Autodesk Inventor part; units mm, degrees
ref_plane "YZ Plane" through (0, 0, 0) normal (1, 0, 0) x (0, 1, 0)
ref_plane "XZ Plane" through (0, 0, 0) normal (0, 1, 0) x (-1, 0, 0)
ref_plane "XY Plane" through (0, 0, 0) normal (0, 0, 1) x (1, 0, 0)
sketch "Эскиз1" plane through (0, 0, 0) normal (0, 0, 1) x (1, 0, 0)
  line L0 (125, -28.5) -> (-125, -28.5)
  line L1 (-125, -28.5) -> (-125, 28.5)
  line L2 (-125, 28.5) -> (125, 28.5)
  line L3 (125, 28.5) -> (125, -28.5)
  line L4 (125, -28.5) -> (-125, 28.5) construction
  line L5 (-125, -28.5) -> (125, 28.5) construction
  line L6 (-125, 28.5) -> (125, 28.5)
  line L7 (125, 11.5) -> (-125, 11.5)
  line L8 (-125, 11.5) -> (-125, 28.5)
  line L9 (-125, 11.5) -> (125, 11.5)
  line L10 (125, 11.5) -> (125, -8.5)
  line L11 (125, -8.5) -> (-125, -8.5)
  line L12 (-125, -8.5) -> (-125, 11.5)
  line L13 (-125, -8.5) -> (125, -8.5)
  line L14 (125, -8.5) -> (125, -25.5)
  line L15 (125, -25.5) -> (-125, -25.5)
  line L16 (-125, -25.5) -> (-125, -8.5)
  line L17 (-125, 28.5) -> (125, 28.5)
  line L18 (125, 25.5) -> (-125, 25.5)
  line L19 (-125, 25.5) -> (-125, 28.5)
  line L20 (-125, 28.5) -> (-111, 28.5)
  line L21 (-111, 28.5) -> (-111, 25.5)
  line L22 (-111, 25.5) -> (-125, 25.5)
  line L23 (-125, 25.5) -> (-125, 28.5)
  line L24 (-111, 25.5) -> (-99, 25.5)
  line L25 (-99, 25.5) -> (-99, 28.5)
  line L26 (-99, 28.5) -> (-111, 28.5)
  line L27 (-111, 28.5) -> (-111, 25.5)
  line L28 (-99, 28.5) -> (-87, 28.5)
  line L29 (-87, 28.5) -> (-87, 25.5)
  line L30 (-87, 25.5) -> (-99, 25.5)
  line L31 (-99, 25.5) -> (-99, 28.5)
  line L32 (-111, 28.5) -> (-106.35, 28.5)
  line L33 (-106.35, 28.5) -> (-103.65, 28.5)
  line L34 (-103.65, 28.5) -> (-103.65, 8.5)
  line L35 (-103.65, 8.5) -> (-106.35, 8.5)
  line L36 (-106.35, 8.5) -> (-106.35, 28.5)
  line L37 (-106.35, 25.5) -> (-107.45, 25.5)
  line L38 (-107.45, 22.5) -> (-106.35, 22.5)
  line L39 (-106.35, 22.5) -> (-106.35, 25.5)
  line L40 (-107.45, 22.5) -> (-102.55, 22.5)
  line L41 (-102.55, 22.5) -> (-102.55, 20.6)
  line L42 (-102.55, 20.6) -> (-107.45, 20.6)
  line L43 (-107.45, 20.6) -> (-107.45, 22.5)
  line L44 (125, -28.5) -> (125, 28.5)
  line L45 (111, 28.5) -> (111, 25.5)
  line L46 (99, 25.5) -> (99, 28.5)
  line L47 (87, 28.5) -> (87, 25.5)
  line L48 (103.65, 28.5) -> (103.65, 8.5)
  line L49 (103.65, 8.5) -> (106.35, 8.5)
  line L50 (106.35, 8.5) -> (106.35, 28.5)
  line L51 (106.35, 22.5) -> (106.35, 25.5)
  line L52 (107.45, 22.5) -> (102.55, 22.5)
  line L53 (102.55, 22.5) -> (102.55, 20.6)
  line L54 (102.55, 20.6) -> (107.45, 20.6)
  line L55 (107.45, 20.6) -> (107.45, 22.5)
  line L56 (-125, 11.5) -> (-96, 11.5)
  line L57 (-96, 11.5) -> (-96, -8.5)
  line L58 (-96, -8.5) -> (-125, -8.5)
  line L59 (-125, -8.5) -> (-125, 11.5)
  line L60 (-96, -8.5) -> (-67, -8.5)
  line L61 (-67, -8.5) -> (-67, 11.5)
  line L62 (-67, 11.5) -> (-96, 11.5)
  line L63 (-96, 11.5) -> (-96, -8.5)
  line L64 (-96, 1.5) -> (-93, 1.5)
  line L65 (-67, 1.5) -> (-70, 1.5)
  circle A0 centre (-70, 1.5) radius 1.5
  circle A1 centre (-93, 1.5) radius 1.5
  circle A2 centre (70, 1.5) radius 1.5
  circle A3 centre (93, 1.5) radius 1.5
  line L66 (-125, 28.5) -> (-122, 28.5)
  line L67 (-126, 8.5) -> (-125, 28.5)
  line L68 (-126, -3.5) -> (-126, 8.5)
  line L69 (-126, 1.15) -> (-126, 3.85)
  line L70 (-125, 28.5) -> (-123, 28.5)
  line L71 (-123, 28.5) -> (-123, 8.5)
  line L72 (-123, 8.5) -> (-125, 8.5)
  line L73 (-125, 8.5) -> (-125, 28.5)
  line L74 (-123, 8.5) -> (-126, 8.5)
  line L75 (-126, 8.5) -> (-126, -3.5)
  line L76 (-126, -3.5) -> (-123, -3.5)
  line L77 (-123, -3.5) -> (-123, 8.5)
  line L78 (-123, 28.5) -> (-120, 28.5)
  line L79 (-120, 28.5) -> (-120, -3.5)
  line L80 (-120, -3.5) -> (-123, -3.5)
  line L81 (-123, -3.5) -> (-123, 28.5)
  line L82 (-123, 8.5) -> (-120, 8.5)
  line L83 (-120, 8.5) -> (-120, -3.5)
  line L84 (-120, -3.5) -> (-123, -3.5)
  line L85 (-123, -3.5) -> (-123, 8.5)
  line L86 (-123, 8.5) -> (-123, 3.85)
  line L87 (-123, 3.85) -> (-103, 3.85)
  line L88 (-103, 3.85) -> (-103, 1.15)
  line L89 (-103, 1.15) -> (-123, 1.15)
  line L90 (-123, 1.15) -> (-123, 3.85)
  line L91 (-120, 1.15) -> (-117, 1.15)
  line L92 (-117, 1.15) -> (-117, 0.05)
  line L93 (-117, 0.05) -> (-120, 0.05)
  line L94 (-120, 0.05) -> (-120, 1.15)
  line L95 (-117, 0.05) -> (-115.1, 0.05)
  line L96 (-115.1, 0.05) -> (-115.1, 4.95)
  line L97 (-115.1, 4.95) -> (-117, 4.95)
  line L98 (-117, 4.95) -> (-117, 0.05)
  line L99 (123, 3.85) -> (103, 3.85)
  line L100 (103, 3.85) -> (103, 1.15)
  line L101 (103, 1.15) -> (123, 1.15)
  line L102 (120, 1.15) -> (117, 1.15)
  line L103 (117, 0.05) -> (115.1, 0.05)
  line L104 (115.1, 0.05) -> (115.1, 4.95)
  line L105 (115.1, 4.95) -> (117, 4.95)
  line L106 (117, 4.95) -> (117, 0.05)
  line L107 (126, -3.5) -> (123, -3.5)
  line L108 (120, 28.5) -> (120, -3.5)
  line L109 (120, -3.5) -> (123, -3.5)
  line L110 (123, -3.5) -> (123, 28.5)
  line L111 (123, 8.5) -> (125, 8.5)
  line L112 (123, 8.5) -> (120, 8.5)
  line L113 (-123, -3.5) -> (-125, -3.5)
  line L114 (-125, -3.5) -> (-125, -28.5)
  line L115 (-125, -28.5) -> (-123, -28.5)
  line L116 (-123, -28.5) -> (-123, -3.5)
  line L117 (123, -3.5) -> (125, -3.5)
  line L118 (125, -3.5) -> (125, -28.5)
  line L119 (125, -28.5) -> (123, -28.5)
  line L120 (123, -28.5) -> (123, -3.5)
  line L121 (-67, -8.5) -> (-14.5, -8.5)
  line L122 (-14.5, -28.5) -> (-67, -28.5)
  line L123 (-40.75, -28.5) -> (-33.75, -28.5)
  circle A4 centre (-33.75, -21.5) radius 1.5
  circle A5 centre (-47.75, -21.5) radius 1.5
  circle A6 centre (33.75, -21.5) radius 1.5
  circle A7 centre (47.75, -21.5) radius 1.5
  line L124 (-33.75, -25.5) -> (-47.75, -25.5)
  line L125 (-47.75, -28.5) -> (-33.75, -28.5)
  line L126 (-40.75, -28.5) -> (-28.75, -28.5)
  line L127 (-28.75, -28.5) -> (-28.75, -25.5)
  line L128 (-28.75, -25.5) -> (-40.75, -25.5)
  line L129 (-40.75, -28.5) -> (-52.75, -28.5)
  line L130 (-52.75, -28.5) -> (-52.75, -25.5)
  line L131 (-52.75, -25.5) -> (-40.75, -25.5)
  line L132 (-40.75, -25.5) -> (-40.75, -28.5)
  line L133 (28.75, -28.5) -> (28.75, -25.5)
  line L134 (52.75, -28.5) -> (52.75, -25.5)
  line L135 (52.5, -17.5) -> (-52.5, -17.5)
  line L136 (-52.5, -17.5) -> (-52.5, 17.5)
  line L137 (-52.5, 17.5) -> (52.5, 17.5)
  line L138 (52.5, 17.5) -> (52.5, -17.5)
  line L139 (52.5, -17.5) -> (-52.5, 17.5) construction
  line L140 (-52.5, -17.5) -> (52.5, 17.5) construction
  line L141 (15, 14.5) -> (-15, 14.5)
  line L142 (-15, 14.5) -> (-15, 20.5)
  line L143 (-15, 20.5) -> (15, 20.5)
  line L144 (15, 20.5) -> (15, 14.5)
  line L145 (15, 14.5) -> (-15, 20.5) construction
  line L146 (-15, 14.5) -> (15, 20.5) construction
  line L147 (15, -20.5) -> (-15, -20.5)
  line L148 (-15, -20.5) -> (-15, -14.5)
  line L149 (-15, -14.5) -> (15, -14.5)
  line L150 (15, -14.5) -> (15, -20.5)
  line L151 (15, -20.5) -> (-15, -14.5) construction
  line L152 (-15, -20.5) -> (15, -14.5) construction
  line L153 (0, 0) -> (-36, 0)
  line L154 (-36, 0) -> (-36, 28.5)
  line L155 (-36, 28.5) -> (0, 28.5)
  line L156 (0, 28.5) -> (0, 0)
  line L157 (0, 0) -> (47, 0)
  line L158 (47, 0) -> (47, 28.5)
  line L159 (47, 28.5) -> (0, 28.5)
  line L160 (0, 28.5) -> (0, 0)
  line L161 (-36, 28.5) -> (-33, 28.5)
  line L162 (-33, 28.5) -> (-33, 25.5)
  line L163 (-33, 25.5) -> (-36, 25.5)
  line L164 (-36, 25.5) -> (-36, 28.5)
  line L165 (-36, 28.5) -> (-39, 28.5)
  line L166 (-39, 28.5) -> (-39, 25.5)
  line L167 (-39, 25.5) -> (-36, 25.5)
  line L168 (-36, 25.5) -> (-36, 28.5)
  line L169 (47, 28.5) -> (44, 28.5)
  line L170 (44, 28.5) -> (44, 25.5)
  line L171 (44, 25.5) -> (47, 25.5)
  line L172 (47, 25.5) -> (47, 28.5)
  line L173 (47, 28.5) -> (50, 28.5)
  line L174 (50, 28.5) -> (50, 25.5)
  line L175 (50, 25.5) -> (47, 25.5)
  line L176 (47, 25.5) -> (47, 28.5)
  line L177 (-39, 25.5) -> (-33, 25.5)
  line L178 (-33, 25.5) -> (-33, 22.5)
  line L179 (-33, 22.5) -> (-39, 22.5)
  line L180 (-39, 22.5) -> (-39, 25.5)
  line L181 (50, 25.5) -> (44, 25.5)
  line L182 (44, 25.5) -> (44, 22.5)
  line L183 (44, 22.5) -> (50, 22.5)
  line L184 (50, 22.5) -> (50, 25.5)
  line L185 (-70, 1.5) -> (70, 1.5)
  line L186 (0, 1.5) -> (10, 1.5)
  line L187 (10, 1.5) -> (-10, 1.5)
  circle A8 centre (-10, 1.5) radius 1.5
  circle A9 centre (10, 1.5) radius 1.5
  point P0 (106.35, 20.6)
  point P1 (103.65, 20.6)
  point P2 (103.65, 22.5)
  point P3 (103.65, 25.5)
  point P4 (-103.65, 25.5)
  point P5 (-103.65, 22.5)
  point P6 (-103.65, 20.6)
  point P7 (-106.35, 20.6)
  point P8 (106.35, 11.5)
  point P9 (103.65, 11.5)
  point P10 (-103.65, 11.5)
  point P11 (-106.35, 11.5)
  point P12 (-120, 3.85)
  point P13 (-117, 3.85)
  point P14 (-115.1, 3.85)
  point P15 (-115.1, 1.15)
  point P16 (-117, 1.15)
  point P17 (-120, 1.15)
  point P18 (115.1, 1.15)
  point P19 (115.1, 3.85)
  point P20 (117, 3.85)
  point P21 (120, 3.85)
  point P22 (120, 11.5)
  point P23 (-123, -28.5)
  point P24 (123, 28.5)
  point P25 (0, 17.5)
  point P26 (0, -17.5)
  point P27 (-15, 17.5)
  point P28 (15, 17.5)
  point P29 (-15, -17.5)
  point P30 (15, -17.5)
  point P31 (-123, -25.5)
  point P32 (123, -25.5)
  dimension "d0" = 250
  dimension "d1" = 57
  dimension "d2" = 17
  dimension "d3" = 20
  dimension "d4" = 17
  dimension "d8" = 3
  dimension "d9" = 14
  dimension "d10" = 12
  dimension "d11" = 12
  dimension "d12" = 4.65
  dimension "d14" = 20
  dimension "d15" = 1.1
  dimension "d16" = 3
  dimension "d17" = 4.9
  dimension "d18" = 1.9
  dimension "d23" = 29
  dimension "d24" = 29
  dimension "d25" = 3
  dimension "d26" = 3
  dimension "d27" = 3
  dimension "d31" = 4.65
  dimension "d37" = 2
  dimension "d38" = 20
  dimension "d39" = 12
  dimension "d40" = 3
  dimension "d41" = 20
  dimension "d42" = 2.7
  dimension "d43" = 3
  dimension "d44" = 1.1
  dimension "d45" = 1.9
  dimension "d46" = 4.9
  dimension "d49" = 3
  dimension "d50" = 12
  dimension "d51" = 12
  dimension "d52" = 105
  dimension "d53" = 35
  dimension "d54" = 30
  dimension "d55" = 6
  dimension "d56" = 30
  dimension "d57" = 6
  dimension "d58" = 33.75
  dimension "d59" = 36
  dimension "d60" = 47
  dimension "d61" = 3
  dimension "d62" = 3
  dimension "d63" = 3
  dimension "d64" = 3
  dimension "d65" = 96
  dimension "d66" = 10
  dimension "d67" = 20
  dimension "d68" = 3
  dimension "d69" = 3
extrude "Выдавливание1" add sketch "Эскиз1" along normal blind 3 contours L15 L116 L11 L136 L135 L148 L147 L150 L138 L120 | L11 L138 L7 L48 L49 L50 L108 L99 L106 L105 L104 L100 L101 L103 L109 L120 | L138 L135 L150 L149 L148 L136 L11 | L11 L136 L185 L154 L153 L157 L158 L138 | L185 L158 L7 L138 | L112 L108 L7 L110 | L11 L61 L185 L136 | L138 L137 L158 L183 L184 L18 L48 L52 L53 L54 L7 | L7 L158 L137 L138 | L185 A9 L156 L7 L158 | L158 L157 A9 L185 | L135 L148 L149 L150 | L7 L108 L18 L110 | L11 L57 L7 L61 | L185 L61 L7 L136 | L136 L7 L154 L185 | L7 L156 L141 L144 L137 L158 | L18 L108 L2 L110 | L7 L50 L54 L55 L52 L18 L108 | L11 L116 L80 L79 L93 L95 L96 L89 L88 L87 L97 L98 L7 L36 L35 L34 L57 | L136 L137 L154 L7 | L7 L34 L42 L41 L40 L18 L180 L179 L154 L137 L136 | L185 A8 L153 L154 | L154 L7 L156 L185 A8 | L7 L154 L137 L142 L141 L156 | L137 L144 L143 L156 L18 L182 L183 L158 | L157 L156 L185 A9 | L18 L45 L2 L108 | L156 L137 L144 L141 | L141 L142 L137 L156 | L156 L153 A8 L185 | L154 L179 L178 L18 L156 L143 L142 L137 | L18 L47 L2 L46 | L89 L92 L93 L79 | L7 L79 L18 L36 L38 L43 L42 | L71 L7 L79 L82 | L7 L71 L18 L79 | L79 L2 L21 L18 | L18 L71 L2 L79 | L18 L25 L2 L29
equation "\"Радиус_гибки\" = Толщина"
equation "\"Ширина_просечки\" = Толщина"
equation "\"Глубина_просечки\" = 0.5 * Толщина"
equation "\"Размер_просечки\" = 4 * Толщина"
equation "\"Мин_остаток\" = 2 * Толщина"
equation "\"Радиус_перехода\" = Радиус_гибки"
equation "\"Радиус_Якоби\" = Радиус_гибки"
equation "\"Размер_зазора\" = Толщина"
properties part number "зад" material "Дерево (орех)"
Read the model definition and answer for the solid it produces. Units are mm, in the model's axes. Coordinates: 2 decimals unless noted, no trailing zeros. Write each loop counter-clockwise with the first axis right and the second up, starting at its lowest first coordinate (ties: lowest second). Pieces come first, ordered by that corner, then holes. Notation, with made-up numbers: (10.25, 6) -> (14.25, 6) arc R20 cw to (14.25, 44) -> close; hole circle Ø7 at (77.5, 47). An arc over 180 degrees is marked (long way). Write item = value, one per line.
(1) Given pin 1 Ø1.2 at (x, z) = (-106.5, 1.5) entering from +Y; pin 2 Ø0.9 at (y, z) = (4.5, 1.5) entering from +X, each flat-ended and moving along its own axis, determine where each tip first touches the part or whether it passes through.
From the geometry:
pin_1 = 25.5
pin_2 = 120
(2) Straight lines are drawn through the part: L1, parallel to Y at x = 107, z = 2.1; L2, parallel to Y at x = -10, z = 0.9; L3, parallel to Y at x = -93, z = 1.7. For each, find the intervals that lie inside material, in ascending order. Write a range as from..to.
From the geometry:
L1 = -25.5..1.15, 3.85..20.6, 22.5..25.5
L2 = -25.5..-20.5, -17.5..0, 3..17.5, 20.5..25.5
L3 = -25.5..0, 3..28.5
(3) Section A-A on z = 0.7 is taken. Count the separate pieces of the cut face and the enclosed holes in it, plus the area to 3 significant figures.
From the geometry:
separate_pieces = 1
enclosed_holes = 12
area = 12,100 mm2
(4) For a pull along Z with two mould halves and no side action, classify faces 1 (the face through (-2, 2, 0)), 2 (the face through (-2, 2, 3)) as +Z half, -Z half, draft (parallel to the pull), parting line (faces both ways), or undercut.
From the geometry:
face_1 = -Z half
face_2 = +Z half
(5) Section B-B on x = 27 is taken. Write down the section's boundary in (y, z), plus the area to 3 significant figures.
From the geometry:
outline = (-25.5, 0) -> (25.5, 0) -> (25.5, 3) -> (-25.5, 3) -> close
area = 153 mm2
